```python
from build123d import *

# Parameters (mm, degrees)
SKETCH_1_R      = 1.6
SKETCH_1_W      = 66
SKETCH_1_H      = 2.5
SKETCH_1_W_2    = 70
SKETCH_1_W_3    = 13
SKETCH_1_H_2    = 9
SKETCH_1_W_4    = 10
SKETCH_1_H_3    = 12
EXTRUDE_1_DEPTH = 1.5
SKETCH_1_3_W    = 70
SKETCH_1_3_H    = 2.5
SKETCH_1_3_W_2  = 66
EXTRUDE_2_DEPTH = 8
SKETCH_1_4_W    = 6.5
SKETCH_1_4_H    = 12
SKETCH_1_4_W_2  = 10
EXTRUDE_3_DEPTH = 11
SKETCH_1_5_W    = 13
SKETCH_1_5_H    = 9
SKETCH_1_5_W_2  = 1
EXTRUDE_4_DEPTH = 11


with BuildPart() as part:
    # Sketch 1 → Extrude 1 (new body)
    # profile 1 of 6: a face of its own
    with BuildSketch(Plane(origin=(0, 0, 0), x_dir=(1, 0, 0), z_dir=(0, 1, 0))):
        Polygon((-22.889699569, -10.997660222), (-22.889699569, -15.497660222), (76.170300431, -15.497660222), (76.170300431, -14.497660222), (78.710300431, -11.957660222), (78.710300431, 23.362339778), (76.170300431, 25.902339778), (76.170300431, 35.302339778), (75.210300431, 36.262339778), (75.210300431, -8.657660222), (70.210300431, -8.657660222), (70.210300431, 37.342339778), (74.130300431, 37.342339778), (73.630300431, 37.842339778), (-22.889699569, 37.842339778), (-22.889699569, 29.842339778), (-12.889699569, 29.842339778), (-12.889699569, 17.842339778), (-22.889699569, 17.842339778), (-22.889699569, -1.997660222), (-9.889699569, -1.997660222), (-9.889699569, -10.997660222), align=None)
        with Locations(Location((-7.649699569, -12.957660222, 0), (0, 0, 270))):
            Circle(SKETCH_1_R, mode=Mode.SUBTRACT)
        with Locations((37.710300431, -13.247660222)):
            Rectangle(SKETCH_1_W, SKETCH_1_H, mode=Mode.SUBTRACT)
        with Locations(Location((73.630300431, -12.957660222, 0), (0, 0, 270))):
            Circle(SKETCH_1_R, mode=Mode.SUBTRACT)
        with Locations(Location((-7.649699569, 35.302339778, 0), (0, 0, 270))):
            Circle(SKETCH_1_R, mode=Mode.SUBTRACT)
        with Locations((30.210300431, 36.092339778)):
            Rectangle(SKETCH_1_W_2, SKETCH_1_H, mode=Mode.SUBTRACT)
        with Locations(Location((67.280300431, 35.302339778, 0), (0, 0, 270))):
            Circle(SKETCH_1_R, mode=Mode.SUBTRACT)
    # profile 2 of 6: a face of its own
    with BuildSketch(Plane(origin=(0, 0, 0), x_dir=(1, 0, 0), z_dir=(0, 1, 0))):
        with Locations((-16.389699569, -6.497660222)):
            Rectangle(SKETCH_1_W_3, SKETCH_1_H_2)
    # profile 3 of 6: a face of its own
    with BuildSketch(Plane(origin=(0, 0, 0), x_dir=(1, 0, 0), z_dir=(0, 1, 0))):
        with Locations((-17.889699569, 23.842339778)):
            Rectangle(SKETCH_1_W_4, SKETCH_1_H_3)
    # profile 4 of 6: a face of its own
    with BuildSketch(Plane(origin=(0, 0, 0), x_dir=(1, 0, 0), z_dir=(0, 1, 0))):
        with Locations((30.210300431, 36.092339778)):
            Rectangle(SKETCH_1_W_2, SKETCH_1_H)
    # profile 5 of 6: a face of its own
    with BuildSketch(Plane(origin=(0, 0, 0), x_dir=(1, 0, 0), z_dir=(0, 1, 0))):
        with Locations((37.710300431, -13.247660222)):
            Rectangle(SKETCH_1_W, SKETCH_1_H)
    # profile 6 of 6: a face of its own
    with BuildSketch(Plane(origin=(0, 0, 0), x_dir=(1, 0, 0), z_dir=(0, 1, 0))):
        Polygon((75.210300431, 36.262339778), (74.130300431, 37.342339778), (70.210300431, 37.342339778), (70.210300431, -8.657660222), (75.210300431, -8.657660222), align=None)
    extrude(amount=-EXTRUDE_1_DEPTH)

    # Sketch 1_3 → Extrude 2 (add)
    with BuildSketch(Plane(origin=(0, 0, 0), x_dir=(1, 0, 0), z_dir=(0, 1, 0))):
        with Locations((30.210300431, 36.092339778)):
            Rectangle(SKETCH_1_3_W, SKETCH_1_3_H)
        Polygon((75.210300431, 36.262339778), (74.130300431, 37.342339778), (70.210300431, 37.342339778), (70.210300431, -8.657660222), (75.210300431, -8.657660222), align=None)
        with Locations((37.710300431, -13.247660222)):
            Rectangle(SKETCH_1_3_W_2, SKETCH_1_3_H)
    extrude(amount=EXTRUDE_2_DEPTH)

    # Sketch 1_4 → Extrude 3 (add)
    with BuildSketch(Plane(origin=(0, 0, 0), x_dir=(1, 0, 0), z_dir=(0, 1, 0))):
        with Locations((-26.139699569, 23.842339778)):
            Rectangle(SKETCH_1_4_W, SKETCH_1_4_H)
        with Locations((-17.889699569, 23.842339778)):
            Rectangle(SKETCH_1_4_W_2, SKETCH_1_4_H)
    extrude(amount=EXTRUDE_3_DEPTH)

    # Sketch 1_5 → Extrude 4 (add)
    with BuildSketch(Plane(origin=(0, 0, 0), x_dir=(1, 0, 0), z_dir=(0, 1, 0))):
        with Locations((-16.389699569, -6.497660222)):
            Rectangle(SKETCH_1_5_W, SKETCH_1_5_H)
        with Locations((-23.389699569, -6.497660222)):
            Rectangle(SKETCH_1_5_W_2, SKETCH_1_5_H)
    extrude(amount=EXTRUDE_4_DEPTH)


solid = part.part
```
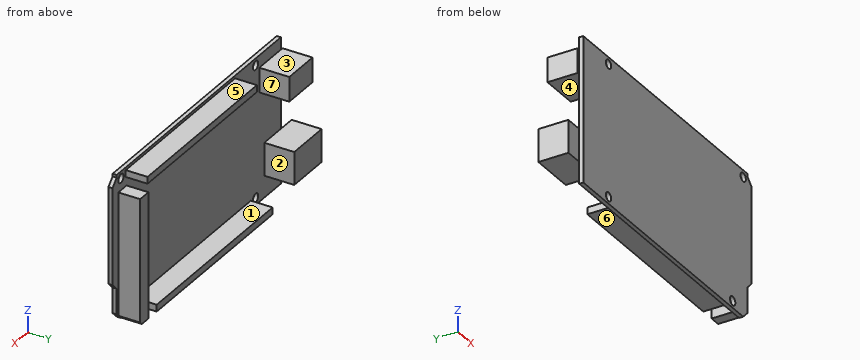
The model under review builds one solid part; all positions refer to its coordinate system, in mm. Face numbers are marked on the shaded views. A direction names the side the tool comes from. Round coordinates to 2 decimals unless told otherwise and drop trailing zeros. Loops run counter-clockwise (first coordinate to the right, second up) from the corner with the lowest first, then second, coordinate; pieces in that order, holes last. Notation, with made-up numbers: M 42.5,75 L 68.5,75 A9 cw 68.5,86 Z; hole C 65,80.25 d3. An arc over 180 degrees is marked long. Put each result on its own line as item: value.
Q1. Consider section A-A, the plane y = 9.75. Give the boundary of the cut face in (x, z), then the cut area to 3 significant figures.
Result set:
outline: M -29.39,-29.84 L -12.89,-29.84 L -12.89,-17.84 L -29.39,-17.84 Z; M -23.89,2 L -9.89,2 L -9.89,11 L -23.89,11 Z
area: 324 mm²
Q2. For pin 1 (5 mm diameter, centred on y = 7, z = -15.5, fed in from +X); pin 2 (5 mm diameter, centred on x = -27.5, z = -25.5, fed in from -Y); pin 3 (3 mm diameter, centred on x = 41, y = 2, fed in from -Z), all flat-tipped, find the tip position at first contact; note any pin that passes through.
Result set:
pin 1: stops at x = 75.21
pin 2: stops at y = 0
pin 3: stops at z = -37.34
Q3. Consider section C-C, the plane z = 10. Give the boundary of the cut face in (x, y), then the cut area to 3 significant figures.
Result set:
outline: M -23.89,0 L -22.89,0 L -22.89,-1.5 L 78.71,-1.5 L 78.71,0 L -9.89,0 L -9.89,11 L -23.89,11 Z
area: 306 mm²
Q4. Consider section D-D, the plane x = -11. Give the boundary of the cut face in (y, z), then the cut area to 3 significant figures.
Result set:
outline: M -1.5,-37.84 L 0,-37.84 L 0,2 L 11,2 L 11,11 L 0,11 L 0,15.5 L -1.5,15.5 Z
area: 179 mm²
Q5. Machinability: for the marked faces 4, 5, 6 and 7, which of the approach directions +Z, -Z, +X, -X, +Y, -Y give a long, thin tool a straight path to every point of the face, cutting with its end or side? Answer none if there is none.
Result set:
face 4: -X, +Y
face 5: +Z, +X, -X, +Y
face 6: -Z, +X, -X, +Y
face 7: +Z, -Z, +Y
Q6. Consider section B-B, the plane y = 3.5. Give the boundary of the cut face in (x, z), then the cut area to 3 significant figures.
Result set:
outline: M -29.39,-29.84 L -12.89,-29.84 L -12.89,-17.84 L -29.39,-17.84 Z; M -23.89,2 L -9.89,2 L -9.89,11 L -23.89,11 Z; M -4.79,-37.34 L 65.21,-37.34 L 65.21,-34.84 L -4.79,-34.84 Z; M 4.71,12 L 70.71,12 L 70.71,14.5 L 4.71,14.5 Z; M 70.21,-37.34 L 74.13,-37.34 L 75.21,-36.26 L 75.21,8.66 L 70.21,8.66 Z
area: 893 mm²
Q7. To check wall thickness, follow L1, parallel to X at y = 6.75, z = 4; L2, parallel to Z at x = 8.5, y = 2.75; L3, parallel to X at y = 3.5, z = -19.5. State the ranges of each line that lie inside material, in increasing order.
Result set:
L1: x = -23.89 to -9.89, 70.21 to 75.21
L2: z = -37.34 to -34.84, 12 to 14.5
L3: x = -29.39 to -12.89, 70.21 to 75.21
Q8. Mouldability with a two-part tool opening along Z and no side actions: class the marked faces 1, 2 and 3 as released by +Z, released by -Z, zero draft, split by the parting line, or undercut.
Result set:
face 1: undercut
face 2: zero draft
face 3: released by +Z
